Verification items for this drawing (mm, ordinates from the low corner). A direction names the side the tool comes from. Give positions to 0.01 mm unless a question says otherwise; leave off trailing zeros. Loops run counter-clockwise (first coordinate to the right, second up) from the corner with the lowest first, then second, coordinate; pieces in that order, holes last. Notation, with made-up numbers: (-8, 56.5) -> (17, 56.5) arc R22 cw to (17, 63.5) -> close; hole circle Ø3 at (59, -35.75). An arc over 180 degrees is marked (long way). Answer in a Markdown table with one row per item. Add a question column.
Q1. Section check A-A on y = 87.5. Enter the section's corners in (x, z), and give its area (3 significant figures).
Q2. Gauge pin test, flat ends, axial feed: P1, Ø5, axis at x = 17.5, z = 38, coming from the +Y side; P2, Ø4.5, axis at x = 57.5, z = 9, coming from the +Y side; P3, Ø17.5, axis at x = 58, z = 32.5, coming from the +Y side. Record the tip position at first contact, or that the pin passes through.
Q3. Release check for a two-part mould opening along X. For the marked faces 6, 7 and 8 record: pulls with the +X half, pulls with the -X half, needs draft (parallel to the pull), parting line crosses it, or undercut.
Q4. Section check C-C on x = 50. Enter the section's corners in (y, z).
Q5. Section check D-D on y = 64.5. Enter the section's corners in (x, z).
Q6. Section check B-B on z = 25.5. Enter the section's corners in (x, y).
Q7. Material ranges on probe 1 along X at (y, z) = (43, 26.5); probe 2 along X at (y, z) = (83, 5.5); probe 3 along X at (y, z) = (36, 36.5), recorded low to high.
Q8. Set-up check for the marked faces 1, 2, 3, 4 and 5: record each of +Z, -Z, +X, -X, +Y, -Y from which the full face is reachable in a straight line by a thin tool's end or side.
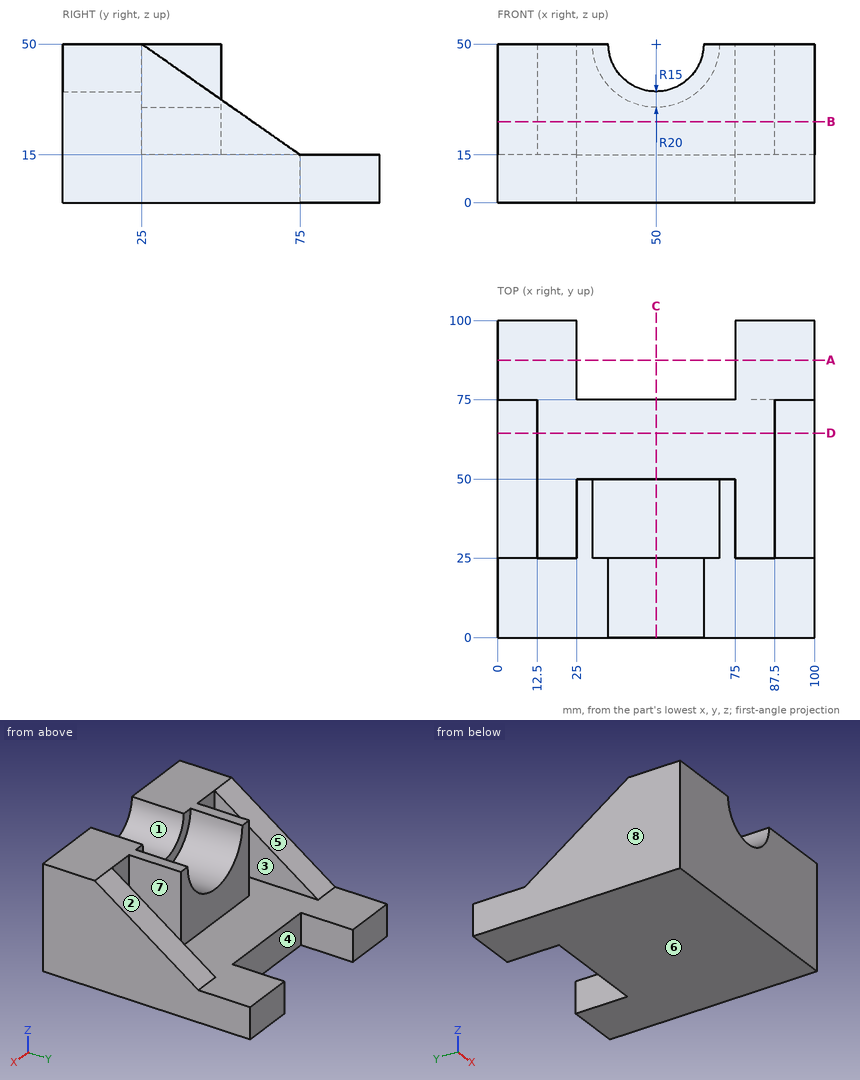
Taken from the geometry:
| question | item | result |
|---|---|---|
| 1 | outline | (0, 0) -> (25, 0) -> (25, 15) -> (0, 15) -> close; (75, 0) -> (100, 0) -> (100, 15) -> (75, 15) -> close |
| 1 | area | 750 mm² |
| 2 | P1 | stops at y = 25 |
| 2 | P2 | stops at y = 75 |
| 2 | P3 | stops at y = 50 |
| 3 | face 6 | needs draft |
| 3 | face 7 | undercut |
| 3 | face 8 | pulls with the -X half |
| 4 | outline | (0, 0) -> (75, 0) -> (75, 15) -> (50, 15) -> (50, 30) -> (25, 30) -> (25, 35) -> (0, 35) -> close |
| 5 | outline | (0, 0) -> (100, 0) -> (100, 22.35) -> (87.5, 22.35) -> (87.5, 15) -> (12.5, 15) -> (12.5, 22.35) -> (0, 22.35) -> close |
| 6 | outline | (0, 0) -> (100, 0) -> (100, 60) -> (87.5, 60) -> (87.5, 25) -> (75, 25) -> (75, 50) -> (25, 50) -> (25, 25) -> (12.5, 25) -> (12.5, 60) -> (0, 60) -> close |
| 7 | probe 1 | x = 0 to 12.5, 25 to 75, 87.5 to 100 |
| 7 | probe 2 | x = 0 to 25, 75 to 100 |
| 7 | probe 3 | x = 0 to 12.5, 25 to 35.24, 64.76 to 75, 87.5 to 100 |
| 8 | face 1 | +Z, +Y, -Y |
| 8 | face 2 | +Z, +X, +Y |
| 8 | face 3 | +Z, +Y |
| 8 | face 4 | +Z, -Z, +Y |
| 8 | face 5 | +Z, -X, +Y |
